```python
from build123d import *

# Parameters (mm, degrees)
F1_DEPTH = 19.05


with BuildPart() as f1:
    # F0 (on Front) → F1 (new body)
    with BuildSketch(Plane.XZ):
        with BuildLine():
            Line((-1.5875, 4.4064), (-1.5875, 6.148361))
            ThreePointArc((-1.5875, 6.148361), (0, -6.35), (1.5875, 6.148361))
            Line((1.5875, 6.148361), (1.5875, 4.4064))
            Line((1.5875, 4.4064), (-1.5875, 4.4064))
        make_face()
        with BuildLine():
            ThreePointArc((-1, -3.872983), (0, 4), (1, -3.872983))
            Line((1, -3.872983), (1, -4.872983))
            Line((1, -4.872983), (-1, -4.872983))
            Line((-1, -4.872983), (-1, -3.872983))
        make_face(mode=Mode.SUBTRACT)
    extrude(amount=F1_DEPTH)


solid = f1.part
```
The model under review builds one solid part; all positions refer to its coordinate system, in mm. A direction names the side the tool comes from. Round coordinates to 2 decimals unless told otherwise and drop trailing zeros. Loops run counter-clockwise (first coordinate to the right, second up) from the corner with the lowest first, then second, coordinate; pieces in that order, holes last.
1) The part is to be moulded in two halves that separate along X. For faces 4 (the face through (1.588, -9, 5)), 5 (the face through (-3, 0, -3)), 6 (the face through (-0.257, -9.392, -6.345)), say which applies: pulls with the +X half, pulls with the -X half, needs draft (parallel to the pull), parting line crosses it, or undercut.
Values follow:
face 4: undercut
face 5: needs draft
face 6: parting line crosses it
2) Consider section D-D on x = -4.25. State the section outline as (y, z) points, then the cut area to 3 significant figures.
Values follow:
outline: (-19.05, -4.72) - (0, -4.72) - (0, 4.72) - (-19.05, 4.72) - close
area: 180 mm2
3) Tool access review of faces 1 (the face through (0, -9, 4.406)), 2 (the face through (-3, -19.05, -3)), 3 (the face through (0, -9, -4.873)): name each direction out of +Z, -Z, +X, -X, +Y, -Y from which nothing blocks a thin tool from reaching the whole face with its end or side.
Values follow:
face 1: +Z, +Y, -Y
face 2: +Z, -Z, +X, -X, -Y
face 3: +Y, -Y
4) Wall thickness on line 1 along X through (y, z) = (-6.5, 0); line 2 along Z through (x, y) = (0.75, -18); line 3 along Z through (x, y) = (0, -10): over which ranges is each line inside the solid? List them lowest first.
Values follow:
line 1: x = -6.35 to -4, 4 to 6.35
line 2: z = -6.31 to -4.87, 3.93 to 4.41
line 3: z = -6.35 to -4.87, 4 to 4.41
5) Consider section C-C on y = -2.75. State the section outline as (x, z) points.
Values follow:
outline: (-1.59, 4.41) - (-1.59, 6.15) arc R6.35 ccw (long way) to (1.59, 6.15) - (1.59, 4.41) - close; hole (-1, -4.87) - (1, -4.87) - (1, -3.87) arc R4 ccw (long way) to (-1, -3.87) - close
6) Consider section A-A on z = 0. State the section outline as (x, y) points, then the cut area to 3 significant figures.
Values follow:
outline: (-6.35, -19.05) - (-4, -19.05) - (-4, 0) - (-6.35, 0) - close; (4, -19.05) - (6.35, -19.05) - (6.35, 0) - (4, 0) - close
area: 89.5 mm2
7) Clearance check with flat-ended pins moving along their axes: P1, Ø1.9, axis at y = -8.5, z = 5, coming from the +X side; P2, Ø1.1, axis at y = -14, z = -4, coming from the +X side; P3, Ø1.9, axis at y = -5.5, z = 5, coming from the -X side; P4, Ø6.5, axis at x = 0, z = 0, coming from the +Y side. State where each tip first meets the part, or that it passes through.
Values follow:
P1: stops at x = 4.89
P2: stops at x = 5.33
P3: stops at x = -4.89
P4: passes through
8) Consider section B-B on x = 0. State the section outline as (y, z) points, then the cut area to 3 significant figures.
Values follow:
outline: (-19.05, -6.35) - (0, -6.35) - (0, -4.87) - (-19.05, -4.87) - close; (-19.05, 4) - (0, 4) - (0, 4.41) - (-19.05, 4.41) - close
area: 35.9 mm2
